Build history of the part. All positions in model axes, mm. A direction names the side the tool comes from. Round coordinates to 2 decimals unless told otherwise and drop trailing zeros. Use a Markdown table: item, result.
from build123d import *

# Parameters (mm, degrees)
BOSS_EXTRUDE2_DEPTH = 6.35


with BuildPart() as part:
    # Sketch1 → Boss-Extrude2 (new body)
    with BuildSketch(Plane.XY):
        with BuildLine():
            Line((-19.05, 0), (-15.24, 1.386726593))
            Line((-15.24, 1.386726593), (-15.24, 0))
            add(Edge.make_bspline(
                [(-15.24, 0), (-13.932101613, -20.478619227), (0, -19.05)],
                knots=[0, 0, 0, 0.635745988, 0.635745988, 0.635745988], degree=2))
            Line((0, -19.05), (-1.386726593, -15.24))
            Line((-1.386726593, -15.24), (0, -15.24))
            add(Edge.make_bspline(
                [(0, -15.24), (20.478619227, -13.932101613), (19.05, 0)],
                knots=[0, 0, 0, 0.635745988, 0.635745988, 0.635745988], degree=2))
            Line((19.05, 0), (15.24, -1.386726593))
            Line((15.24, -1.386726593), (15.24, 0))
            add(Edge.make_bspline(
                [(15.24, 0), (13.932101613, 20.478619227), (0, 19.05)],
                knots=[0, 0, 0, 0.635745988, 0.635745988, 0.635745988], degree=2))
            Line((0, 19.05), (1.386726593, 15.24))
            Line((1.386726593, 15.24), (0, 15.24))
            add(Edge.make_bspline(
                [(0, 15.24), (-20.478619227, 13.932101613), (-19.05, 0)],
                knots=[0, 0, 0, 0.635745988, 0.635745988, 0.635745988], degree=2))
        make_face()
        with BuildLine():
            Line((6.594985068, -2.811017562), (6.613082013, 2.810596285))
            ThreePointArc((6.613082013, 2.810596285), (7.502999025, 4.342309614), (5.731905154, 4.305915826))
            Line((5.731905154, 4.305915826), (0.872493224, 7.132395163))
            ThreePointArc((0.872493224, 7.132395163), (-0.009050924, 8.668942567), (-0.863079915, 7.116933388))
            Line((-0.863079915, 7.116933388), (-5.740588789, 4.321798878))
            ThreePointArc((-5.740588789, 4.321798878), (-7.512049949, 4.326632954), (-6.594985068, 2.811017562))
            Line((-6.594985068, 2.811017562), (-6.613082013, -2.810596285))
            ThreePointArc((-6.613082013, -2.810596285), (-7.502999025, -4.342309614), (-5.731905154, -4.305915826))
            Line((-5.731905154, -4.305915826), (-0.872493224, -7.132395163))
            ThreePointArc((-0.872493224, -7.132395163), (0.009050924, -8.668942567), (0.863079915, -7.116933388))
            Line((0.863079915, -7.116933388), (5.740588789, -4.321798878))
            ThreePointArc((5.740588789, -4.321798878), (7.512049949, -4.326632954), (6.594985068, -2.811017562))
        make_face(mode=Mode.SUBTRACT)
    extrude(amount=BOSS_EXTRUDE2_DEPTH)


solid = part.part
Q1. Drill centre lines: L1, parallel to X at y = 7.5, z = 2.5; L2, parallel to Y at x = -3, z = 3.5; L3, parallel to X at y = -8, z = 1. Where is each one in solid material? Low to high.
Response values:
| item | result |
|---|---|
| L1 | x = -17.79 to -1, 1 to 14.17 |
| L2 | y = -19.09 to -5.89, 5.89 to 14.97 |
| L3 | x = -14.04 to -0.95, 0.95 to 17.5 |
Q2. Drop flat-ended pins along their axis: P1, Ø1.5, axis at y = -12, z = 1.5, coming from the +X side; P2, Ø12, axis at x = -10.5, y = 15, coming from the +Z side; P3, Ø2, axis at y = -12.5, z = 3, coming from the -X side; P4, Ø1.1, axis at y = 1, z = 3, coming from the -X side. Give the stop position or say it passes through.
Response values:
| item | result |
|---|---|
| P1 | stops at x = 14.37 |
| P2 | stops at z = 6.35 |
| P3 | stops at x = -12.84 |
| P4 | stops at x = -19.14 |
Q3. Two-plate mould, pull along Y, no slides. Class faces 5 (the flat face through (-17.172, 0.684, 3.131)), 6 (the cylindrical face through (7.5, -4.35, 3.13)), 7 (the flat face through (17.172, -0.684, 3.131)), 8 (the flat face through (9, 0, 6.35)): +Y half, -Y half, draft (parallel to the pull), parting line (faces both ways), or undercut.
Response values:
| item | result |
|---|---|
| face 5 | -Y half |
| face 6 | undercut |
| face 7 | +Y half |
| face 8 | draft |
Q4. Which spindle directions (+Z, -Z, +X, -X, +Y, -Y) get a long thin tool onto all of the face, cutting with end or side? Do faces 1 (the flat face through (15.24, -1, 3)), 2 (the flat face through (-1, -15.24, 3)), 3 (the flat face through (0.684, 17.172, 3.131)), 4 (the flat face through (3.336, 5.699, 3.131)). Say none if no direction does.
Response values:
| item | result |
|---|---|
| face 1 | +Z, -Z, +Y |
| face 2 | +Z, -Z, +X |
| face 3 | +Z, -Z, -X |
| face 4 | +Z, -Z |
